Here's how the part is built. I have some questions about the finished solid (model axes, mm). A direction names the side the tool comes from. Round coordinates to 2 decimals unless told otherwise and drop trailing zeros. Write each loop counter-clockwise with the first axis right and the second up, starting at its lowest first coordinate (ties: lowest second). Pieces come first, ordered by that corner, then holes. Notation, with made-up numbers: (80.5, 66) - (91.5, 66) arc R17 ccw to (91.5, 83) - close; hole circle Ø10 at (36, 6). An arc over 180 degrees is marked (long way). Use one line per item in the form item = value. Start each with the question number.
1. If I drill on line 1 along X through (y, z) = (-16, 9.75); line 2 along X through (y, z) = (12.5, 0); line 3 along Y through (x, z) = (-6.25, -8.5), over which ranges is the centre line in solid material (lowest first)?
2. I want a section at B-B, the plane y = -15. List the corners of the cut face in (x, z) for me, plus the area to 3 significant figures.
3. Which directions (+Z, -Z, +X, -X, +Y, -Y) give clear straight access to the entire face, cutting with the end or side of a thin tool? Please do faces 5 (the cylindrical face through (-13.339, -17.625, 0.151)), 6 (the flat face through (0, 0, 10)).
4. I want a section at D-D, the plane y = 17. List the corners of the cut face in (x, z) for me, plus the area to 3 significant figures.
5. I want a section at A-A, the plane x = 0. List the corners of the cut face in (y, z) for me.
6. Will these pins go through, and if not, where does the flat tip stop? pin 1 (10 mm diameter, centred on x = -0.5, y = 21.5, fed in from -Z); pin 2 (1.5 mm diameter, centred on y = 2.5, z = 8.5, fed in from +X); pin 3 (6 mm diameter, centred on x = 3.5, z = 0.5, fed in from -Y).
7. I want a section at C-C, the plane z = 0. List the corners of the cut face in (x, y) for me (3 decimals), plus the area to 3 significant figures.
8. We'd pull the mould along Z, two halves only. Please class faces 1 (the flat face through (0, 0, 0)), 2 (the cylindrical face through (14.4, -0.57, 0.15)), 3 (the cylindrical face through (5.78, 8.11, -7.54)), 4 (the cylindrical face through (-1.88, 13.31, 5.96)): +Z half, -Z half, draft (parallel to the pull), parting line (faces both ways), or undercut.
```python
from build123d import *

# Parameters (mm, degrees)
BOSS_EXTRUDE1_DEPTH = 10.75
FILLET2_R           = 2


with BuildPart() as part:
    # Sketch1 → Boss-Extrude1 (new, symmetric)
    with BuildSketch(Plane.XY):
        with BuildLine():
            Line((-13, 0), (13, 0))
            ThreePointArc((13, 0), (14.414213562, -0.585786438), (15, -2))
            Line((15, -2), (15, -16))
            ThreePointArc((15, -16), (13.375, -17.625), (11.75, -16))
            ThreePointArc((11.75, -16), (0, -4.25), (-11.75, -16))
            ThreePointArc((-11.75, -16), (-13.375, -17.625), (-15, -16))
            Line((-15, -16), (-15, -2))
            ThreePointArc((-15, -2), (-14.414213562, -0.585786438), (-13, 0))
        make_face()
    extrude(amount=BOSS_EXTRUDE1_DEPTH, both=True)

    # Sketch3 → Revolve1 (revolve)
    with BuildSketch(Plane.XY, mode=Mode.PRIVATE) as revolve1_sk:
        Polygon((-9.5, 0), (-9.5, 16), (-8.537624701, 27), (-6.25, 27), (-6.25, 0), align=None)
    revolve(revolve1_sk.sketch.rotate(Axis((0, 13.186129828, 0), (0, -1, 0)), 270), axis=Axis((0, 13.186129828, 0), (0, -1, 0)))

    # Fillet2
    fillet2_edges = [part.edges().sort_by_distance(p)[0] for p in [
        (0, 27, -8.537624701),
    ]]
    fillet(fillet2_edges, radius=FILLET2_R)


solid = part.part
```
Model answer:
q1.line_1 = -15 to -11.75, 11.75 to 15
q1.line_2 = -9.5 to -6.25, 6.25 to 9.5
q1.line_3 = -6.05 to 0
q2.outline = (-15, -10.75) - (-11.71, -10.75) - (-11.71, 10.75) - (-15, 10.75) - close; (11.71, -10.75) - (15, -10.75) - (15, 10.75) - (11.71, 10.75) - close
q2.area = 142 mm2
q3.face_5 = +Z, -Z, -Y
q3.face_6 = +Y
q4.outline = circle Ø18.83 at (0, 0); hole circle Ø12.5 at (0, 0)
q4.area = 156 mm2
q5.outline = (-4.25, -10.75) - (0, -10.75) - (0, -9.5) - (16, -9.5) - (25.17, -8.7) arc R2 ccw to (27, -6.7) - (27, -6.25) - (0, -6.25) - (0, 6.25) - (27, 6.25) - (27, 6.7) arc R2 ccw to (25.17, 8.7) - (16, 9.5) - (0, 9.5) - (0, 10.75) - (-4.25, 10.75) - close
q6.pin_1 = -9.45
q6.pin_2 = 5.49
q6.pin_3 = -6.21
q7.outline = (-15, -16) arc R1.625 ccw to (-11.75, -16) arc R11.75 cw to (11.75, -16) arc R1.625 ccw to (15, -16) - (15, -2) arc R2 ccw to (13, 0) - (9.5, 0) - (9.5, 16) - (8.697, 25.174) arc R2 ccw to (6.705, 27) - (6.25, 27) - (6.25, 0) - (-6.25, 0) - (-6.25, 27) - (-6.705, 27) arc R2 ccw to (-8.697, 25.174) - (-9.5, 16) - (-9.5, 0) - (-13, 0) arc R2 ccw to (-15, -2) - close
q7.area = 433 mm2
q8.face_1 = undercut
q8.face_2 = draft
q8.face_3 = parting line
q8.face_4 = undercut
